Geometry check sheet. Reference: the model listing, model coordinates, mm. Face numbers are marked on the shaded views. A direction names the side the tool comes from. Coordinates: 2 decimals unless noted, no trailing zeros. Write each loop counter-clockwise with the first axis right and the second up, starting at its lowest first coordinate (ties: lowest second). Pieces come first, ordered by that corner, then holes. Notation, with made-up numbers: (22, -6) -> (49, -6) arc R12 ccw to (49, 2) -> close; hole circle Ø3 at (53.25, -30). An arc over 180 degrees is marked (long way). Use a Markdown table: item, result.
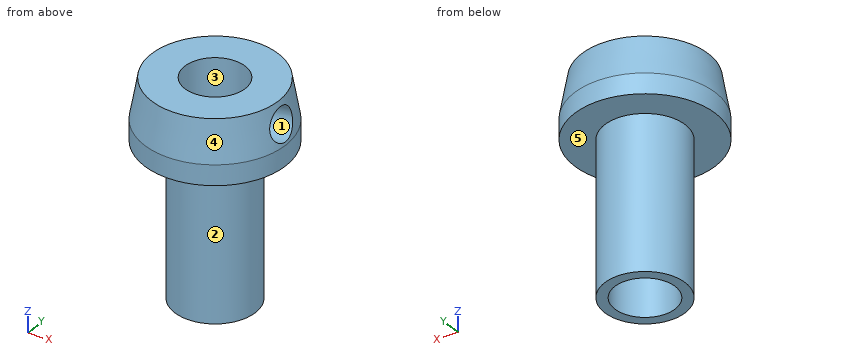
Autodesk Inventor part; units mm, degrees
ref_plane "Work Plane1" through (15.7367, 0, 53) normal (0.9848, 0, 0.1736) x (0, 1, 0)
ref_plane "YZ Plane" through (0, 0, 0) normal (1, 0, 0) x (0, 1, 0)
ref_plane "XY Plane" through (0, 0, 0) normal (0, 0, 1) x (1, 0, 0)
sketch "Sketch1" plane through (0, 0, 0) normal (0, 0, 1) x (1, 0, 0)
  circle A0 centre (0, 0) radius 10
  dimension "d0" = 20
extrude "Extrusion1" add sketch "Sketch1" along normal blind 38
sketch "Sketch2" plane through (0, 0, 38) normal (0, 0, 1) x (1, 0, 0)
  circle A0 centre (0, 0) radius 17.5
  dimension "d3" = 35
extrude "Extrusion2" add sketch "Sketch2" along normal blind 5
sketch "Sketch3" plane through (0, 0, 43) normal (0, 0, 1) x (1, 0, 0)
  circle A0 centre (0, 0) radius 17.5
extrude "Extrusion3" add sketch "Sketch3" along normal blind 10 draft -10
sketch "Sketch4" plane through (0, 0, 53) normal (0, 0, 1) x (1, 0, 0)
  circle A0 centre (0, 0) radius 7.5
  dimension "d9" = 15
extrude "Extrusion4" cut sketch "Sketch4" against normal through all
ref_plane "Work Plane1" through (15.7367, 0, 53) normal (0.9848, 0, 0.1736) x (0, 1, 0)
sketch "Sketch6" plane through (15.7367, 0, 53) normal (0.9848, 0, 0.1736) x (0, 1, 0)
  circle A0 centre (0, -5.4313) radius 4
  point P0 (0, -49.4622)
  dimension "d12" = 8
extrude "Extrusion5" cut sketch "Sketch6" against normal blind 13.25
properties part number "Midle"
Item 1: Mould release check, pull along X, two halves, no side actions. Record for the marked faces 3, 4 and 5: +X half, -X half, draft (parallel to the pull), parting line (faces both ways), or undercut.
Answer block:
| item | result |
|---|---|
| face 3 | undercut |
| face 4 | parting line |
| face 5 | draft |
Item 2: Section check C-C on z = 8.5. Record the boundary of the cut face in (x, y), then the cut area to 3 significant figures.
Answer block:
| item | result |
|---|---|
| outline | circle Ø20 at (0, 0); hole circle Ø15 at (0, 0) |
| area | 137 mm^2 |
Item 3: Section check B-B on y = 0. Record the boundary of the cut face in (x, z).
Answer block:
| item | result |
|---|---|
| outline | (-17.5, 38) -> (-10, 38) -> (-10, 0) -> (-7.5, 0) -> (-7.5, 53) -> (-15.74, 53) -> (-17.5, 43) -> close; (7.5, 0) -> (10, 0) -> (10, 38) -> (17.5, 38) -> (17.5, 43) -> (17.37, 43.71) -> (7.5, 41.97) -> close; (7.5, 50.09) -> (15.99, 51.59) -> (15.74, 53) -> (7.5, 53) -> close |
Item 4: Tool access check on the marked faces 1 and 2. Record the directions out of +Z, -Z, +X, -X, +Y, -Y that give a thin tool (end or side, any length) a straight path to the whole face; none if there is none.
Answer block:
| item | result |
|---|---|
| face 1 | none |
| face 2 | -Z |
Item 5: Section check A-A on x = 0. Record the boundary of the cut face in (y, z), then the cut area to 3 significant figures.
Answer block:
| item | result |
|---|---|
| outline | (-17.5, 38) -> (-10, 38) -> (-10, 0) -> (-7.5, 0) -> (-7.5, 53) -> (-15.74, 53) -> (-17.5, 43) -> close; (7.5, 0) -> (10, 0) -> (10, 38) -> (17.5, 38) -> (17.5, 43) -> (15.74, 53) -> (7.5, 53) -> close |
| area | 472 mm^2 |
Item 6: Thickness scan on L1, parallel to Y at x = 0, z = 17.5; L2, parallel to Y at x = 0, z = 42.5; L3, parallel to Z at x = -10.5, y = 3. Record the ranges inside material, lowest first. Write a range as [from, to].
Answer block:
| item | result |
|---|---|
| L1 | y = [-10, -7.5], [7.5, 10] |
| L2 | y = [-17.5, -7.5], [7.5, 17.5] |
| L3 | z = [38, 53] |
Item 7: Section check D-D on z = 39. Record the boundary of the cut face in (x, y).
Answer block:
| item | result |
|---|---|
| outline | circle Ø35 at (0, 0); hole circle Ø15 at (0, 0) |
Item 8: Depth check by flat-ended pin: P1, Ø2, axis at x = -4.5, y = 7.5, coming from the -Z side; P2, Ø4, axis at x = 7.5, z = 11.5, coming from the +Y side; P3, Ø12, axis at y = -7, z = 13, coming from the +X side; P4, Ø5, axis at y = 5.5, z = 23.5, coming from the -X side. Enter the tip coordinate at first touch or a pass-through.
Answer block:
| item | result |
|---|---|
| P1 | stops at z = 0 |
| P2 | stops at y = 8.35 |
| P3 | stops at x = 9.95 |
| P4 | stops at x = -9.54 |
